Verification items for this drawing (mm, ordinates from the low corner). Give positions to 0.01 mm unless a question says otherwise; leave off trailing zeros. Order: outer loops, then holes, each group sorted by start corner. A loop starts at its lowest first (then second) coordinate and runs counter-clockwise, first axis right, second up. Notation, with made-up numbers: (28.5, -5) - (43.5, -5) arc R15 ccw to (43.5, 12) - close; hole circle Ø5 at (19, 58). An arc over 180 degrees is marked (long way). Put each result on its own line as item: value. Start each with the question number.
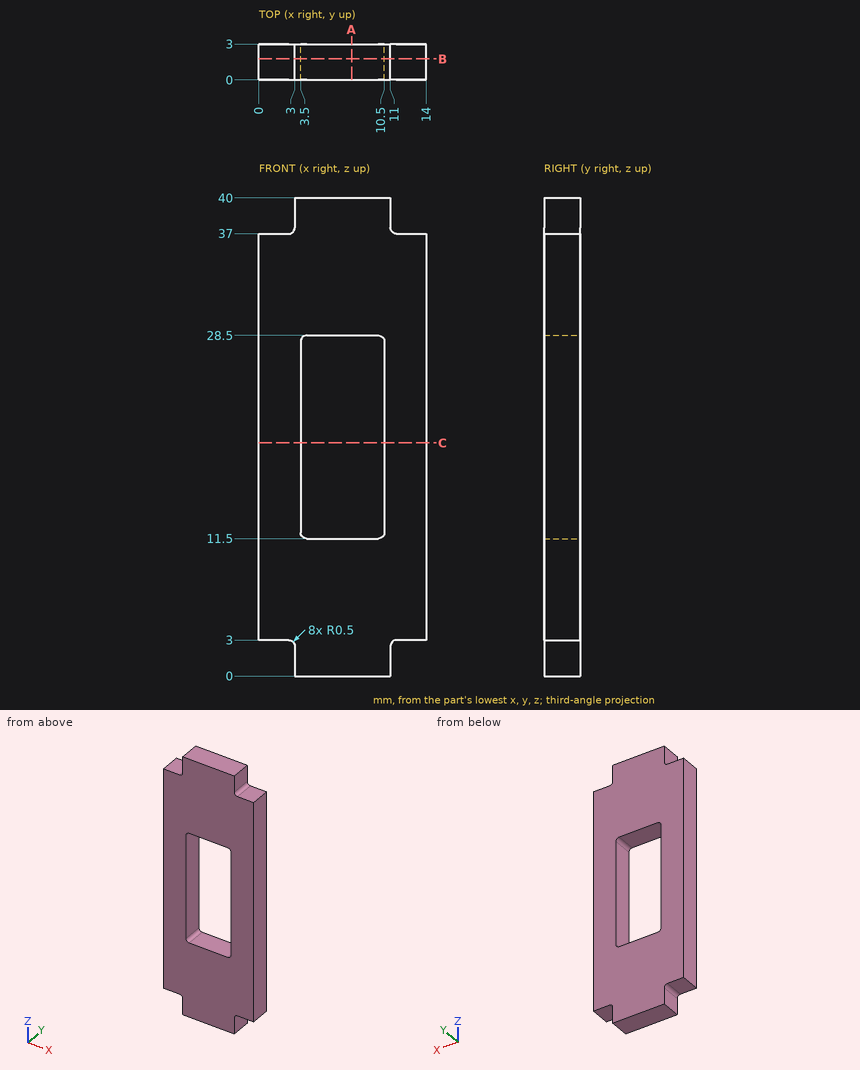
Item 1: Cross-section at C-C (z = 19.5). Enter the section's corners in (x, y).
Item 2: Cross-section at B-B (y = 1.75). Enter the section's corners in (x, z), and give its area (3 significant figures).
Item 3: Cross-section at A-A (x = 7.75). Enter the section's corners in (y, z), and give its area (3 significant figures).
Item 4: Thickness scan on line 1 along Z through (x, y) = (10, 0.45); line 2 along X through (y, z) = (1.1, 26); line 3 along Z through (x, y) = (13, 1.7). Record the ranges inside material, lowest first.
Item 5: Gauge pin test, flat ends, axial feed: pin 1 Ø8 at (x, z) = (7.5, 19) entering from -Y; pin 2 Ø0.8 at (y, z) = (2, 2) entering from -X; pin 3 Ø0.8 at (y, z) = (1.5, 38.5) entering from +X. Record the tip position at first contact, or that the pin passes through.
Recorded:
1. outline: (0, 0) - (3.5, 0) - (3.5, 3) - (0, 3) - close; (10.5, 0) - (14, 0) - (14, 3) - (10.5, 3) - close
2. outline: (0, 3) - (2.5, 3) arc R0.5 cw to (3, 2.5) - (3, 0) - (11, 0) - (11, 2.5) arc R0.5 cw to (11.5, 3) - (14, 3) - (14, 37) - (11.5, 37) arc R0.5 cw to (11, 37.5) - (11, 40) - (3, 40) - (3, 37.5) arc R0.5 cw to (2.5, 37) - (0, 37) - close; hole (3.5, 12) arc R0.5 ccw to (4, 11.5) - (10, 11.5) arc R0.5 ccw to (10.5, 12) - (10.5, 28) arc R0.5 ccw to (10, 28.5) - (4, 28.5) arc R0.5 ccw to (3.5, 28) - close
2. area: 405 mm^2
3. outline: (0, 0) - (3, 0) - (3, 11.5) - (0, 11.5) - close; (0, 28.5) - (3, 28.5) - (3, 40) - (0, 40) - close
3. area: 69.0 mm^2
4. line 1: z = 0 to 11.5, 28.5 to 40
4. line 2: x = 0 to 3.5, 10.5 to 14
4. line 3: z = 3 to 37
5. pin 1: stops at y = 0
5. pin 2: stops at x = 3
5. pin 3: stops at x = 11
